Part model, mm, in its own coordinate system. Round coordinates to 2 decimals unless told otherwise and drop trailing zeros. Write each loop counter-clockwise with the first axis right and the second up, starting at its lowest first coordinate (ties: lowest second). Pieces come first, ordered by that corner, then holes.
```python
from build123d import *

# Parameters (mm, degrees)
F1_DEPTH = 16.4
F3_DEPTH = 12.5
F4_R     = 2.575
F5_DEPTH = 4


with BuildPart() as f1:
    # F0 (on Front) → F1 (new body)
    with BuildSketch(Plane.XZ):
        Polygon((-9.470071, 0), (0, 0), (9.470071, 0), (11.4, 2.3), (0, 2.3), (-11.4, 2.3), align=None)
    extrude(amount=F1_DEPTH)

    # F2 (on Right) → F3 (cut, symmetric)
    with BuildSketch(Plane.YZ):
        Polygon((-2.741004, 0), (0, 0), (0, 2.299975), align=None)
        Polygon((-13.658996, 0), (-16.4, 2.299975), (-16.4, 0), align=None)
    extrude(amount=F3_DEPTH, both=True, mode=Mode.SUBTRACT)

    # F4 (on face) → F5 (join)
    with BuildSketch(Plane.XY.offset(2.3)):
        with Locations((0, -8.2)):
            Circle(F4_R)
    extrude(amount=-F5_DEPTH)


solid = f1.part
```
Q1. Wall check: L1, parallel to Z at x = -7.75, y = -5.5; L2, parallel to X at y = -8.25, z = -0.6; L3, parallel to Y at x = -5.5, z = 1.15. Give the ranges that are in metal, low to high.
Values follow:
L1: z = 0 to 2.3
L2: x = -2.57 to 2.57
L3: y = -15.03 to -1.37
Q2. Cut at B-B on y = -8.2. Write the cut outline in (x, z) (3 decimals), plus the area to 3 significant figures.
Values follow:
outline: (-11.4, 2.3) - (-9.47, 0) - (-2.575, 0) - (-2.575, -1.7) - (2.575, -1.7) - (2.575, 0) - (9.47, 0) - (11.4, 2.3) - close
area: 56.8 mm2
Q3. Cut at C-C on z = -0.4. Write the cut outline in (x, y) (3 decimals), plus the area to 3 significant figures.
Values follow:
outline: circle Ø5.15 at (0, -8.2)
area: 20.8 mm2
Q4. Mould opens along Z. For faces 1 (the flat face through (0, -8, -1.7)), 2 (the flat face through (0, -8, 2.3)), 3 (the cylindrical face through (-0.558, -10.714, -0.838)) say: +Z half, -Z half, draft (parallel to the pull), parting line (faces both ways), or undercut.
Values follow:
face 1: -Z half
face 2: +Z half
face 3: draft
Q5. Drop flat-ended pins along their axis: pin 1 (1 mm diameter, centred on x = 2, z = -1, fed in from -Y); pin 2 (5 mm diameter, centred on x = 1, y = -13.5, fed in from -Z). Give the stop position or say it passes through.
Values follow:
pin 1: stops at y = -10.29
pin 2: stops at z = 0
